Here's how the part is built. I have some questions about the finished solid (model axes, mm). Face numbers are marked on the shaded views. A direction names the side the tool comes from. Give positions to 0.01 mm unless a question says otherwise; leave off trailing zeros. Order: outer loops, then holes, each group sorted by start corner. A loop starts at its lowest first (then second) coordinate and runs counter-clockwise, first axis right, second up. Notation, with made-up numbers: M 14.5,-34 L 70.5,-34 A25 ccw 70.5,-21 Z; hole C 28,66 d8. An arc over 180 degrees is marked long. Use one line per item in the form item = value.
from build123d import *

# Parameters (mm, degrees)
SKETCH1_W           = 49.9
SKETCH1_H           = 49.9
SKETCH1_W_2         = 19.9
SKETCH1_H_2         = 19.9
BOSS_EXTRUDE1_DEPTH = 15
CHAMFER1_SIZE       = 13.5
CHAMFER2_SIZE       = 13.5
FILLET1_R           = 3.5
SKETCH2_R           = 3
SKETCH2_R_2         = 1.75
CUT_EXTRUDE1_DEPTH  = 3
SKETCH2_2_R         = 1.75
CUT_EXTRUDE2_DEPTH  = 39.34064423
CUT_EXTRUDE3_START  = -1.5
SKETCH3_R           = 1.75
CUT_EXTRUDE3_DEPTH  = 1.5


with BuildPart() as part:
    # Sketch1 → Boss-Extrude1 (new body)
    # profile 1 of 6: a face of its own
    with BuildSketch(Plane(origin=(0, 0, 0), x_dir=(1, 0, 0), z_dir=(0, 1, 0))):
        Rectangle(SKETCH1_W, SKETCH1_H)
        Rectangle(SKETCH1_W_2, SKETCH1_H_2, mode=Mode.SUBTRACT)
    # profile 2 of 6: a face of its own
    with BuildSketch(Plane(origin=(0, 0, 0), x_dir=(1, 0, 0), z_dir=(0, 1, 0))):
        Polygon((-9.95, 9.95), (-9.95, 8.535786438), (-1.414213562, 0), (0, 1.414213562), (-8.535786438, 9.95), align=None)
    # profile 3 of 6: a face of its own
    with BuildSketch(Plane(origin=(0, 0, 0), x_dir=(1, 0, 0), z_dir=(0, 1, 0))):
        Polygon((0, -1.414213562), (8.535786438, -9.95), (9.95, -9.95), (9.95, -8.535786438), (1.414213562, 0), align=None)
    # profile 4 of 6: a face of its own
    with BuildSketch(Plane(origin=(0, 0, 0), x_dir=(1, 0, 0), z_dir=(0, 1, 0))):
        Polygon((0, 1.414213562), (1.414213562, 0), (9.95, 8.535786438), (9.95, 9.95), (8.535786438, 9.95), align=None)
    # profile 5 of 6: a face of its own
    with BuildSketch(Plane(origin=(0, 0, 0), x_dir=(1, 0, 0), z_dir=(0, 1, 0))):
        Polygon((-9.95, -8.535786438), (-9.95, -9.95), (-8.535786438, -9.95), (0, -1.414213562), (-1.414213562, 0), align=None)
    # profile 6 of 6: a face of its own
    with BuildSketch(Plane(origin=(0, 0, 0), x_dir=(1, 0, 0), z_dir=(0, 1, 0))):
        Polygon((-1.414213562, 0), (0, -1.414213562), (1.414213562, 0), (0, 1.414213562), align=None)
    extrude(amount=BOSS_EXTRUDE1_DEPTH)

    # Chamfer1
    chamfer1_edges = [part.edges().sort_by_distance(p)[0] for p in [
        (0, 0, -24.95),
        (24.95, 0, 0),
        (0, 0, 24.95),
        (-24.95, 0, 0),
    ]]
    chamfer(chamfer1_edges, length=CHAMFER1_SIZE)

    # Chamfer2
    chamfer2_edges = [part.edges().sort_by_distance(p)[0] for p in [
        (9.95, 15, 0),
        (0, 15, 9.95),
        (-9.95, 15, 0),
        (0, 15, -9.95),
    ]]
    chamfer(chamfer2_edges, length=CHAMFER2_SIZE)

    # Fillet1
    fillet1_edges = [part.edges().sort_by_distance(p)[0] for p in [
        (0, 7.5, -1.414213562),
        (-1.414213562, 7.5, 0),
        (0, 7.5, 1.414213562),
        (1.414213562, 7.5, 0),
    ]]
    fillet(fillet1_edges, radius=FILLET1_R)

    # Sketch2 → Cut-Extrude1 (cut)
    with BuildSketch(Plane(origin=(0, 15, 0), x_dir=(1, 0, 0), z_dir=(0, 1, 0))):
        Circle(SKETCH2_R)
        with Locations(Location((0, 0, 0), (0, 0, 270))):
            Circle(SKETCH2_R_2, mode=Mode.SUBTRACT)
    extrude(amount=-CUT_EXTRUDE1_DEPTH, mode=Mode.SUBTRACT)

    # Sketch2_2 → Cut-Extrude2 (cut, through all)
    with BuildSketch(Plane(origin=(0, 15, 0), x_dir=(1, 0, 0), z_dir=(0, 1, 0))):
        with Locations(Location((0, 0, 0), (0, 0, 270))):
            Circle(SKETCH2_2_R)
    extrude(amount=-CUT_EXTRUDE2_DEPTH, mode=Mode.SUBTRACT)

    # Sketch3 → Cut-Extrude3 (cut)
    with BuildSketch(Plane.XZ.offset(CUT_EXTRUDE3_START)):
        with BuildLine():
            Line((-8.535786438, 9.95), (-9.95, 9.95))
            Line((-9.95, 9.95), (-9.95, 8.535786438))
            Line((-9.95, 8.535786438), (-3.889087297, 2.474873734))
            ThreePointArc((-3.889087297, 2.474873734), (-2.863961031, 0), (-3.889087297, -2.474873734))
            Line((-3.889087297, -2.474873734), (-9.95, -8.535786438))
            Line((-9.95, -8.535786438), (-9.95, -9.95))
            Line((-9.95, -9.95), (-8.535786438, -9.95))
            Line((-8.535786438, -9.95), (-2.474873734, -3.889087297))
            ThreePointArc((-2.474873734, -3.889087297), (0, -2.863961031), (2.474873734, -3.889087297))
            Line((2.474873734, -3.889087297), (8.535786438, -9.95))
            Line((8.535786438, -9.95), (9.95, -9.95))
            Line((9.95, -9.95), (9.95, -8.535786438))
            Line((9.95, -8.535786438), (3.889087297, -2.474873734))
            ThreePointArc((3.889087297, -2.474873734), (2.863961031, 0), (3.889087297, 2.474873734))
            Line((3.889087297, 2.474873734), (9.95, 8.535786438))
            Line((9.95, 8.535786438), (9.95, 9.95))
            Line((9.95, 9.95), (8.535786438, 9.95))
            Line((8.535786438, 9.95), (2.474873734, 3.889087297))
            ThreePointArc((2.474873734, 3.889087297), (0, 2.863961031), (-2.474873734, 3.889087297))
            Line((-2.474873734, 3.889087297), (-8.535786438, 9.95))
        make_face()
        with Locations(Location((0, 0, 0), (0, 0, 90))):
            Circle(SKETCH3_R, mode=Mode.SUBTRACT)
    extrude(amount=CUT_EXTRUDE3_DEPTH, mode=Mode.SUBTRACT)


solid = part.part
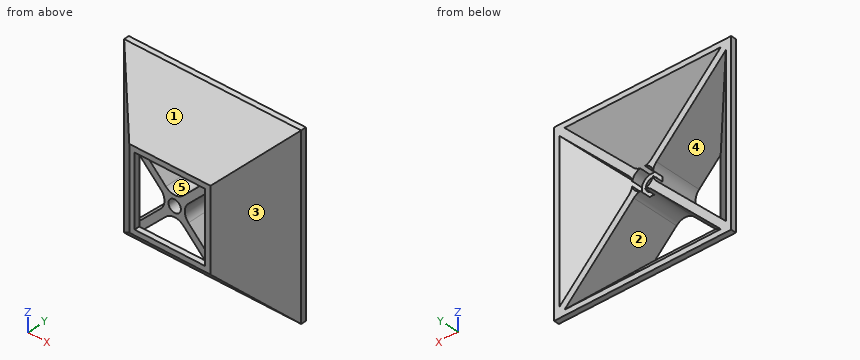
Q1. I'm going to push flat-ended pins straight in: pin 1 Ø0.8 at (x, y) = (0, 1) entering from +Z; pin 2 Ø6 at (x, z) = (4, -1) entering from -Y; pin 3 Ø3 at (y, z) = (4.5, 3.5) entering from -X. Where does each tip first touch, or does it pass through?
Found:
pin_1 = 12.85
pin_2 = 1.5
pin_3 = -17.45
Q2. I need wall thicknesses on L1, parallel to Z at x = 7.5, y = 11.5; L2, parallel to X at y = 8.5, z = 0; L3, parallel to X at y = 12, z = 16. Which ranges of each line are inside material? Lowest first, please.
Found:
L1 = -22.95 to -19.95, -8.91 to -6.09, 6.09 to 8.91, 19.95 to 22.95
L2 = -19.95 to -16.95, -2.86 to -1.75, 1.75 to 2.86, 16.95 to 19.95
L3 = -23.45 to -20.45, -17.41 to -14.59, 14.59 to 17.41, 20.45 to 23.45
Q3. I want a section at D-D on x = 18. Write out the boundary of the cut face in (y, z), then the cut area to 3 significant figures.
Found:
outline = M 6.55,-18 L 13.5,-24.95 L 15,-24.95 L 15,-23.45 L 10.96,-19.41 L 15,-19.41 L 15,-16.59 L 9.55,-16.59 L 9.55,16.59 L 15,16.59 L 15,19.41 L 10.96,19.41 L 15,23.45 L 15,24.95 L 13.5,24.95 L 6.55,18 Z
area = 176 mm²
Q4. Thinking about a two-plate mould opening in X: for the marked faces 1, 2 and 3, which applies, +X half, -X half, draft (parallel to the pull), parting line (faces both ways), or undercut?
Found:
face_1 = draft
face_2 = undercut
face_3 = +X half
Q5. On a 3-axis mill with a long thin cutter (end or side, diameter ignored), from which of +Z, -Z, +X, -X, +Y, -Y can I reach the whole of each face in a straight line? I mean the marked faces 4 and 5. Say none if no direction works.
Found:
face_4 = +Y
face_5 = +Y, -Y
Q6. I want a section at C-C on y = 3. Write out the boundary of the cut face in (x, z), then the cut area to 3 significant figures.
Found:
outline = M -14.45,-14.45 L 14.45,-14.45 L 14.45,14.45 L -14.45,14.45 Z; hole M -11.45,-10.04 L -3.89,-2.47 A3.5 ccw -3.89,2.47 L -11.45,10.04 Z; hole M -10.04,-11.45 L 10.04,-11.45 L 2.47,-3.89 A3.5 ccw -2.47,-3.89 Z; hole M -10.04,11.45 L -2.47,3.89 A3.5 ccw 2.47,3.89 L 10.04,11.45 Z; hole C 0,0 d3.5; hole M 3.89,-2.47 L 11.45,-10.04 L 11.45,10.04 L 3.89,2.47 A3.5 ccw Z
area = 433 mm²
Q7. I want a section at B-B on z = 0. Write out the boundary of the cut face in (x, y).
Found:
outline = M -24.95,13.5 L -11.45,0 L -9.95,0 L -9.95,1.5 L -23.45,15 L -24.95,15 Z; M -2.86,1.5 L -1.75,1.5 L -1.75,12 L -2.86,12 Z; M 1.75,1.5 L 2.86,1.5 L 2.86,12 L 1.75,12 Z; M 9.95,0 L 11.45,0 L 24.95,13.5 L 24.95,15 L 23.45,15 L 9.95,1.5 Z
Q8. I want a section at A-A on x = 0. Write out the boundary of the cut face in (y, z), then the cut area to 3 significant figures.
Found:
outline = M 0,-11.45 L 13.5,-24.95 L 15,-24.95 L 15,-23.45 L 1.5,-9.95 L 0,-9.95 Z; M 0,9.95 L 1.5,9.95 L 15,23.45 L 15,24.95 L 13.5,24.95 L 0,11.45 Z; M 1.5,-2.86 L 12,-2.86 L 12,-1.75 L 1.5,-1.75 Z; M 1.5,1.75 L 12,1.75 L 12,2.86 L 1.5,2.86 Z
area = 109 mm²
